from build123d import *

# Parameters (mm, degrees)
SKETCH_1_W             = 80
SKETCH_1_H             = 40
SM_BASE_FLANGE_1_DEPTH = 3
OTHER_START            = -3
OTHER_1_DEPTH          = 3
HOLE_WIZARD_M8_1_D     = 6.8
HOLE_WIZARD_M10_1_D    = 8.5


# Read off the part's stored shape, not the designer's step: 断开-边角1
# Sheet-metal steps are written as plain solids
with BuildPart() as part:
    # Sketch 1 → 基体-法兰1 (new body)
    with BuildSketch(Plane.XY):
        Rectangle(SKETCH_1_W, SKETCH_1_H)
    extrude(amount=-SM_BASE_FLANGE_1_DEPTH)

    # Other 1 outline → Other 1 (cut)
    with BuildSketch(Plane.XY.offset(OTHER_START)):
        with BuildLine():
            ThreePointArc((40, -15.5), (38.681980515, -18.681980515), (35.5, -20))
            Line((35.5, -20), (40, -20))
            Line((40, -20), (40, -15.5))
        make_face()
        with BuildLine():
            Line((-40, -20), (-35.5, -20))
            ThreePointArc((-35.5, -20), (-38.681980515, -18.681980515), (-40, -15.5))
            Line((-40, -15.5), (-40, -20))
        make_face()
        with BuildLine():
            ThreePointArc((35.5, 20), (38.681980515, 18.681980515), (40, 15.5))
            Line((40, 15.5), (40, 20))
            Line((40, 20), (35.5, 20))
        make_face()
        with BuildLine():
            Line((-40, 20), (-40, 15.5))
            ThreePointArc((-40, 15.5), (-38.681980515, 18.681980515), (-35.5, 20))
            Line((-35.5, 20), (-40, 20))
        make_face()
    extrude(amount=OTHER_1_DEPTH, mode=Mode.SUBTRACT)

    # M8 螺纹孔1 (through all)
    with Locations(Plane.XY):
        with Locations((-20, 0), (20, 0)):
            Hole(HOLE_WIZARD_M8_1_D / 2)

    # M10 螺纹孔1 (through all)
    with Locations(Plane.XY):
        with Locations((0, 0)):
            Hole(HOLE_WIZARD_M10_1_D / 2)


solid = part.part
Geometry: final body of the model. Coordinates: model frame, mm. Give positions to 0.01 mm unless a question says otherwise; leave off trailing zeros. Write each loop counter-clockwise with the first axis right and the second up, starting at its lowest first coordinate (ties: lowest second). Pieces come first, ordered by that corner, then holes. Notation, with made-up numbers: (69.5, 60.25) - (117.5, 60.25) arc R14 ccw to (117.5, 81.25) - close; hole circle Ø7 at (-25.5, 30.5). An arc over 180 degrees is marked (long way). Return JSON: item names as keys, results as strings. Group by question number.
1) Section A-A on x = 0. Return the cut outline in (y, z), plus the area to 3 significant figures.
2) Section D-D on y = -2. Return the cut outline in (x, z), plus the area to 3 significant figures.
3) Section B-B on z = -1.9. Return the cut outline in (x, y), plus the area to 3 significant figures.
4) Mould query, pull axis Y, two halves, no side actions, for faces 1 (the flat face through (-1, 5, -3)), 2 (the cylindrical face through (16.86, -1.3, -1.52)), 3 (the flat face through (0, 20, -1)). Classes: released by +Y, released by -Y, zero draft, split by the parting line, or undercut.
5) Section C-C on x = -20. Return the cut outline in (y, z).
6) Line query: line 1 (Y direction, x = -20, z = -0.7); line 2 (X direction, y = -2, z = -2.7); line 3 (X direction, y = 1.5, z = -1.55). Output: solid intervals per line, ascending.
Filled in:
{
 "1": {"outline": "(-20, -3) - (-4.25, -3) - (-4.25, 0) - (-20, 0) - close; (4.25, -3) - (20, -3) - (20, 0) - (4.25, 0) - close", "area": "94.5 mm^2"},
 "2": {"outline": "(-40, -3) - (-22.75, -3) - (-22.75, 0) - (-40, 0) - close; (-17.25, -3) - (-3.75, -3) - (-3.75, 0) - (-17.25, 0) - close; (3.75, -3) - (17.25, -3) - (17.25, 0) - (3.75, 0) - close; (22.75, -3) - (40, -3) - (40, 0) - (22.75, 0) - close", "area": "185 mm^2"},
 "3": {"outline": "(-40, -15.5) arc R4.5 ccw to (-35.5, -20) - (35.5, -20) arc R4.5 ccw to (40, -15.5) - (40, 15.5) arc R4.5 ccw to (35.5, 20) - (-35.5, 20) arc R4.5 ccw to (-40, 15.5) - close; hole circle Ø6.8 at (-20, 0); hole circle Ø8.5 at (0, 0); hole circle Ø6.8 at (20, 0)", "area": "3,050 mm^2"},
 "4": {"face 1": "zero draft", "face 2": "undercut", "face 3": "released by +Y"},
 "5": {"outline": "(-20, -3) - (-3.4, -3) - (-3.4, 0) - (-20, 0) - close; (3.4, -3) - (20, -3) - (20, 0) - (3.4, 0) - close"},
 "6": {"line 1": "y = -20 to -3.4, 3.4 to 20", "line 2": "x = -40 to -22.75, -17.25 to -3.75, 3.75 to 17.25, 22.75 to 40", "line 3": "x = -40 to -23.05, -16.95 to -3.98, 3.98 to 16.95, 23.05 to 40"}
}
